Could you check a few things on this model? Use its own coordinates, in mm. A direction names the side the tool comes from. Coordinates: 2 decimals unless noted, no trailing zeros. Order: outer loops, then holes, each group sorted by start corner. A loop starts at its lowest first (then second) coordinate and runs counter-clockwise, first axis right, second up. Notation, with made-up numbers: (50.25, 73.25) -> (77.25, 73.25) arc R21 ccw to (77.25, 85.25) -> close; hole circle Ø8 at (29.25, 48). An arc over 180 degrees is marked (long way). Put each result on its own line as item: value. Start each with the question number.
Q1. If we section it at D-D (x = 7): Please give me the cut outline in (y, z), and give its area (3 significant figures).
Q2. Please list where these lines run through material, in increasing order: line 1 along Y through (x, z) = (6.5, 3.65); line 2 along X through (y, z) = (2.75, 0.85); line 3 along X through (y, z) = (1.5, 3.55).
Q3. We'd pull the mould along X, two halves only. Please class faces 1 (the face through (-6, 0, 2)), 2 (the face through (7.727, 0.249, 2.378)), 3 (the face through (19, 0, 2)): +X half, -X half, draft (parallel to the pull), parting line (faces both ways), or undercut.
Q4. If we section it at C-C (z = 1.65): Please give me the cut outline in (x, y), and give its area (3 significant figures).
Q5. If we section it at A-A (y = 0): Please give me the cut outline in (x, z), and give its area (3 significant figures).
Q6. If we section it at B-B (y = 2): Please give me the cut outline in (x, z).
Q7. Will this pin go through, and if not, where does the flat tip stop? pin 1 (2 mm diameter, centred on y = 1.5, z = 2, fed in from +X).
Q8. For faces 4 (the face through (-4.22, -1.24, 2.38)), 5 (the face through (-0.739, 1.597, 0.394)), which set-ups out of +Z, -Z, +X, -X, +Y, -Y let a thin tool reach every point of the face, with its end or its side?
from build123d import *

# Parameters (mm, degrees)
F1_DEPTH = 4
F2_DEPTH = 0.8


# Not quite as in the source:
# - a feature names something its author has since deleted; it is built from what else it names


with BuildPart() as f1:
    # F0 (on Top) → F1 (new body)
    with BuildSketch(Plane.XY):
        with BuildLine():
            Line((8.4610678831, 6), (0, 6))
            ThreePointArc((0, 6), (-6, 0), (0, -6))
            Line((0, -6), (0.6982972488, -6))
            Line((0.6982972488, -6), (0, -4.4))
            ThreePointArc((0, -4.4), (-4.2440131224, -1.1611858666), (-2.2400400253, 3.7871124469))
            Line((-2.2400400253, 3.7871124469), (13, -4.4))
            Line((13, -4.4), (3.8406348682, -4.4))
            Line((3.8406348682, -4.4), (4.5389321169, -6))
            Line((4.5389321169, -6), (13, -6))
            ThreePointArc((13, -6), (19, 0), (13, 6))
            Line((13, 6), (12.3017027512, 6))
            Line((12.3017027512, 6), (13, 4.4))
            ThreePointArc((13, 4.4), (17.2440131224, 1.1611858666), (15.2400400253, -3.7871124469))
            Line((15.2400400253, -3.7871124469), (0, 4.4))
            Line((0, 4.4), (9.1593651318, 4.4))
            Line((9.1593651318, 4.4), (8.4610678831, 6))
        make_face()
    extrude(amount=F1_DEPTH)

    # F0 (on Top) → F2 (join)
    with BuildSketch(Plane.XY):
        with BuildLine():
            ThreePointArc((-2.2400400253, 3.7871124469), (-4.2440131224, -1.1611858666), (0, -4.4))
            Line((0, -4.4), (-0.8065333223, -2.552))
            Line((-0.8065333223, -2.552), (-1.6130666446, -0.704))
            ThreePointArc((-1.6130666446, -0.704), (-0.704, 1.6130666446), (1.6130666446, 0.704))
            Line((1.6130666446, 0.704), (3.8406348682, -4.4))
            Line((3.8406348682, -4.4), (13, -4.4))
            Line((13, -4.4), (-2.2400400253, 3.7871124469))
        make_face()
        with BuildLine():
            Line((11.3869333554, -0.704), (9.1593651318, 4.4))
            Line((9.1593651318, 4.4), (0, 4.4))
            Line((0, 4.4), (15.2400400253, -3.7871124469))
            ThreePointArc((15.2400400253, -3.7871124469), (17.2440131224, 1.1611858666), (13, 4.4))
            Line((13, 4.4), (14.6130666446, 0.704))
            ThreePointArc((14.6130666446, 0.704), (13.704, -1.6130666446), (11.3869333554, -0.704))
        make_face()
    extrude(amount=F2_DEPTH)


solid = f1.part
The answers:
1. outline: (-6, 0) -> (6, 0) -> (6, 4) -> (4.4, 4) -> (4.4, 0.8) -> (0.64, 0.8) -> (0.64, 4) -> (-1.18, 4) -> (-1.18, 0.8) -> (-4.4, 0.8) -> (-4.4, 4) -> (-6, 4) -> close
1. area: 25.7 mm^2
2. line 1: -6 to -4.4, -0.91 to 0.91, 4.4 to 6
2. line 2: -5.33 to -3.43, -0.31 to 3.07, 16.43 to 18.33
2. line 3: -5.81 to -4.14, 2.02 to 5.4, 17.14 to 18.81
3. face 1: -X half
3. face 2: undercut
3. face 3: +X half
4. outline: (-2.24, 3.79) -> (13, -4.4) -> (3.84, -4.4) -> (4.54, -6) -> (13, -6) arc R6 ccw to (13, 6) -> (12.3, 6) -> (13, 4.4) arc R4.4 cw to (15.24, -3.79) -> (0, 4.4) -> (9.16, 4.4) -> (8.46, 6) -> (0, 6) arc R6 ccw to (0, -6) -> (0.7, -6) -> (0, -4.4) arc R4.4 cw to start
4. area: 110 mm^2
5. outline: (-6, 0) -> (-1.76, 0) -> (-1.76, 0.8) -> (-4.4, 0.8) -> (-4.4, 4) -> (-6, 4) -> close; (1.92, 0) -> (11.08, 0) -> (11.08, 0.8) -> (8.19, 0.8) -> (8.19, 4) -> (4.81, 4) -> (4.81, 0.8) -> (1.92, 0.8) -> close; (14.76, 0) -> (19, 0) -> (19, 4) -> (17.4, 4) -> (17.4, 0.8) -> (14.76, 0.8) -> close
5. area: 35.2 mm^2
6. outline: (-5.66, 0) -> (10.21, 0) -> (10.21, 0.8) -> (4.47, 0.8) -> (4.47, 4) -> (1.09, 4) -> (1.09, 0.8) -> (-3.92, 0.8) -> (-3.92, 4) -> (-5.66, 4) -> close; (14.05, 0) -> (18.66, 0) -> (18.66, 4) -> (16.92, 4) -> (16.92, 0.8) -> (14.05, 0.8) -> close
7. pin 1: x = 18.98
8. face 4: +Z
8. face 5: +Z, -Z
